```python
from build123d import *

# Parameters (mm, degrees)
SKETCH1_W               = 36
SKETCH1_H               = 9
BOSS_EXTRUDE1_DEPTH     = 28
CUT_EXTRUDE1_DEPTH      = 28
CUT_EXTRUDE2_DEPTH      = 36
SKETCH5_W               = 11.440376565
SKETCH5_H               = 15.618965423
CUT_EXTRUDE4_DEPTH      = 2
CUT_EXTRUDE5_DEPTH      = 2
CUT_EXTRUDE5_DEPTH_BACK = 2
CUT_EXTRUDE6_DEPTH      = 26
CUT_EXTRUDE7_DEPTH      = 26
SKETCH10_R              = 3
CUT_EXTRUDE8_DEPTH      = 7
SKETCH11_R              = 1.5
CUT_EXTRUDE9_DEPTH      = 2
SKETCH12_R              = 1.5
CUT_EXTRUDE10_DEPTH     = 9
SKETCH13_W              = 5.3
SKETCH13_H              = 5.3
CUT_EXTRUDE11_DEPTH     = 2.5


with BuildPart() as part:
    # Sketch1 → Boss-Extrude1 (new body)
    with BuildSketch(Plane.XY):
        with Locations((18, 4.5)):
            Rectangle(SKETCH1_W, SKETCH1_H)
    extrude(amount=BOSS_EXTRUDE1_DEPTH)

    # Sketch2 → Cut-Extrude1 (cut)
    with BuildSketch(Plane.XY):
        Polygon((0, 4.5), (4.5, 9), (0, 9), align=None)
        Polygon((36, 4.5), (31.5, 9), (36, 9), align=None)
    extrude(amount=CUT_EXTRUDE1_DEPTH, mode=Mode.SUBTRACT)

    # Sketch3 → Cut-Extrude2 (cut)
    with BuildSketch(Plane(origin=(0, 0, 0), x_dir=(0, 0, -1), z_dir=(1, 0, 0))):
        Polygon((-28, 4.5), (-23.5, 9), (-28, 9), align=None)
    extrude(amount=CUT_EXTRUDE2_DEPTH, mode=Mode.SUBTRACT)

    # Sketch5 → Cut-Extrude4 (cut)
    with BuildSketch(Plane(origin=(32, 0, 32), x_dir=(0, 1, 0), z_dir=(0.707106781, 0, 0.707106781))):
        with Locations((5.720188283, -5.935696583)):
            Rectangle(SKETCH5_W, SKETCH5_H)
    extrude(amount=-CUT_EXTRUDE4_DEPTH, mode=Mode.SUBTRACT)

    # Sketch6 → Cut-Extrude5 (cut, two sides)
    with BuildSketch(Plane(origin=(4, 0, -4), x_dir=(0.577350269, -0.577350269, 0.577350269), z_dir=(-0.707106781, 0, 0.707106781))) as cut_extrude5_sk:
        Polygon((26.558112383, 29.802125204), (32.719347855, 28.647424665), (30.19862658, 32.212262879), align=None)
    extrude(amount=CUT_EXTRUDE5_DEPTH, mode=Mode.SUBTRACT)
    extrude(cut_extrude5_sk.sketch, amount=-CUT_EXTRUDE5_DEPTH_BACK, mode=Mode.SUBTRACT)

    # Sketch7 → Cut-Extrude6 (cut)
    with BuildSketch(Plane.XY):
        Polygon((5, 0), (5, 3), (5.707106781, 3.707106781), (13.104524105, 3.707106781), (13.811630886, 3), (13.811630886, 0), align=None)
    extrude(amount=CUT_EXTRUDE6_DEPTH, mode=Mode.SUBTRACT)

    # Sketch8 → Cut-Extrude7 (cut)
    with BuildSketch(Plane.XY.offset(28)):
        Polygon((36, 0), (30, 0), (34.5, 4.5), (34.5, 6), (36, 6), align=None)
    extrude(amount=-CUT_EXTRUDE7_DEPTH, mode=Mode.SUBTRACT)

    # Sketch10 → Cut-Extrude8 (cut)
    with BuildSketch(Plane(origin=(0, 9, 0), x_dir=(1, 0, 0), z_dir=(0, 1, 0))):
        with Locations((22, -6.5)):
            Circle(SKETCH10_R)
    extrude(amount=-CUT_EXTRUDE8_DEPTH, mode=Mode.SUBTRACT)

    # Sketch11 → Cut-Extrude9 (cut)
    with BuildSketch(Plane(origin=(0, 2, 0), x_dir=(1, 0, 0), z_dir=(0, 1, 0))):
        with Locations((22, -6.5)):
            Circle(SKETCH11_R)
    extrude(amount=-CUT_EXTRUDE9_DEPTH, mode=Mode.SUBTRACT)

    # Sketch12 → Cut-Extrude10 (cut)
    with BuildSketch(Plane(origin=(0, 0, 0), x_dir=(1, 0, 0), z_dir=(0, 1, 0))):
        with Locations((22, -16.5)):
            Circle(SKETCH12_R)
    extrude(amount=CUT_EXTRUDE10_DEPTH, mode=Mode.SUBTRACT)

    # Sketch13 → Cut-Extrude11 (cut)
    with BuildSketch(Plane(origin=(0, 9, 0), x_dir=(1, 0, 0), z_dir=(0, 1, 0))):
        with Locations((22, -16.5)):
            Rectangle(SKETCH13_W, SKETCH13_H)
    extrude(amount=-CUT_EXTRUDE11_DEPTH, mode=Mode.SUBTRACT)


solid = part.part
```
Design review of the part built by this model. Coordinates are the model's own, in mm. A direction names the side the tool comes from. Give positions to 0.01 mm unless a question says otherwise; leave off trailing zeros. Order: outer loops, then holes, each group sorted by start corner. A loop starts at its lowest first (then second) coordinate and runs counter-clockwise, first axis right, second up. Notation, with made-up numbers: (57, 50) - (84, 50) arc R28 cw to (84, 79) - close; hole circle Ø8 at (12, 73.5). An arc over 180 degrees is marked (long way). Use a Markdown table: item, result. Add a question column.
(1) Add section D-D on x = 8.5. Give the boundary of the cut face in (y, z).
(2) Add section A-A on z = 6.5. Give the boundary of the cut face in (x, y).
(3) Wall thickness on probe 1 along Z at (x, y) = (22, 2.5); probe 2 along Z at (x, y) = (22, 1.2); probe 3 along X at (y, z) = (1.1, 6.5): over which ranges is each line inside the solid? List them lowest first. Write a range as [from, to].
(4) Add section C-C on x = 22. Give the boundary of the cut face in (y, z).
(5) Machinability: for faces 1 (the face through (9, 2, 26)), 2 (the face through (34, 2, 2)), 3 (the face through (24.65, 8, 17)), which of the approach directions +Z, -Z, +X, -X, +Y, -Y give a long, thin tool a straight path to every point of the face, cutting with its end or side? Answer none if there is none.
(6) Add section B-B on y = 1.5. Give the boundary of the cut face in (x, z), then the cut area to 3 significant figures.
(7) Clearance check with flat-ended pins moving along their axes: P1, Ø7, axis at x = 22, z = 6.5, coming from the +Y side; P2, Ø3, axis at x = 22, y = 8, coming from the +Z side; P3, Ø1.9, axis at x = 8.5, y = 2.5, coming from the -Z side; P4, Ø1.6, axis at y = 5.5, z = 14, coming from the +X side. State where each tip first meets the part, or that it passes through.
(8) Mouldability with a two-part tool opening along X and no side actions: class faces 4 (the face through (22, 8, 13.85)), 5 (the face through (34.5, 5, 15)), 6 (the face through (16.4, 6.7, 25.8)) as +X half, -X half, draft (parallel to the pull), parting line (faces both ways), or undercut.
Report:
| question | item | result |
|---|---|---|
| 1 | outline | (0, 26) - (3.71, 26) - (3.71, 0) - (9, 0) - (9, 23.5) - (4.5, 28) - (0, 28) - close |
| 2 | outline | (0, 0) - (5, 0) - (5, 3) - (5.71, 3.71) - (13.1, 3.71) - (13.81, 3) - (13.81, 0) - (20.5, 0) - (20.5, 2) - (19, 2) - (19, 9) - (4.5, 9) - (0, 4.5) - close; (23.5, 0) - (30, 0) - (34.5, 4.5) - (34.5, 6) - (31.5, 9) - (25, 9) - (25, 2) - (23.5, 2) - close |
| 3 | probe 1 | z = [0, 3.5], [9.5, 15], [18, 28] |
| 3 | probe 2 | z = [0, 5], [8, 15], [18, 28] |
| 3 | probe 3 | x = [0, 5], [13.81, 20.5], [23.5, 31.1] |
| 4 | outline | (0, 0) - (9, 0) - (9, 3.5) - (2, 3.5) - (2, 5) - (0, 5) - close; (0, 8) - (2, 8) - (2, 9.5) - (9, 9.5) - (9, 13.85) - (6.5, 13.85) - (6.5, 15) - (0, 15) - close; (0, 18) - (6.5, 18) - (6.5, 19.15) - (9, 19.15) - (9, 23.5) - (4.5, 28) - (0, 28) - close |
| 5 | face 1 | -Z, -Y |
| 5 | face 2 | +Z, +X, -Y |
| 5 | face 3 | +Y |
| 6 | outline | (0, 0) - (5, 0) - (5, 26) - (13.81, 26) - (13.81, 0) - (36, 0) - (36, 2) - (31.5, 2) - (31.5, 28) - (0, 28) - close; hole circle Ø3 at (22, 6.5); hole circle Ø3 at (22, 16.5) |
| 6 | area | 648 mm² |
| 7 | P1 | stops at y = 9 |
| 7 | P2 | stops at z = 26 |
| 7 | P3 | stops at z = 26 |
| 7 | P4 | stops at x = 34.5 |
| 8 | face 4 | undercut |
| 8 | face 5 | +X half |
| 8 | face 6 | draft |
